from build123d import *

# Parameters (mm, degrees)
BOSS_EXTRUDE1_DEPTH             = 25
SKETCH2_R                       = 1.55
CUT_EXTRUDE1_DEPTH              = 17.55
BOSS_EXTRUDE2_REACH             = 68.8
BOSS_EXTRUDE2_DIRECTION_2_DEPTH = 30
CUT_EXTRUDE2_REACH              = 80.634
CUT_EXTRUDE2_END_RADIUS         = 15.55
SKETCH7_R                       = 1.55


with BuildPart() as part:
    # Sketch1 → Boss-Extrude1 (new, symmetric)
    with BuildSketch(Plane.XY):
        with BuildLine():
            Line((-20.55, 17.55), (-20.55, 0))
            Line((-20.55, 0), (20.55, 0))
            Line((20.55, 0), (20.55, 17.55))
            Line((20.55, 17.55), (12.55, 17.55))
            ThreePointArc((12.55, 17.55), (0, 5), (-12.55, 17.55))
            Line((-12.55, 17.55), (-20.55, 17.55))
        make_face()
    extrude(amount=BOSS_EXTRUDE1_DEPTH, both=True)

    # Sketch2 → Cut-Extrude1 (cut)
    with BuildSketch(Plane(origin=(0, 17.55, 0), x_dir=(1, 0, 0), z_dir=(0, 1, 0))):
        with Locations(Location((-16.55, 15, 0), (0, 0, 270))):
            Circle(SKETCH2_R)
        with Locations(Location((16.55, 15, 0), (0, 0, 270))):
            Circle(SKETCH2_R)
        with Locations(Location((16.55, -15, 0), (0, 0, 270))):
            Circle(SKETCH2_R)
        with Locations(Location((-16.55, -15, 0), (0, 0, 270))):
            Circle(SKETCH2_R)
    extrude(amount=-CUT_EXTRUDE1_DEPTH, mode=Mode.SUBTRACT)

    # Boss-Extrude2: up to this plane
    boss_extrude2_end = Plane(origin=(20.55, 0, 25), z_dir=(-1, 0, 0))
    # Sketch5 → Boss-Extrude2 (add, up to the surface)
    with BuildSketch(Plane(origin=(28.704083189, 0, 16.572310156), x_dir=(0.500000000000001, 0, -0.8660254037844382), z_dir=(0.866025403784438, 0, 0.5000000000000009)), mode=Mode.PRIVATE) as boss_extrude2_sk1:
        with BuildLine():
            Line((-5.334622532, 17.55), (-2.314823147, 17.55))
            ThreePointArc((-2.314823147, 17.55), (10.235176853, 5), (22.785176853, 17.55))
            Line((22.785176853, 17.55), (25.765377468, 17.55))
            ThreePointArc((25.765377468, 17.55), (10.215377468, 2), (-5.334622532, 17.55))
        make_face()
    boss_extrude2_tool1 = split(extrude(boss_extrude2_sk1.sketch, amount=-BOSS_EXTRUDE2_REACH, mode=Mode.PRIVATE), bisect_by=boss_extrude2_end, keep=Keep.BOTH, mode=Mode.PRIVATE)
    add(boss_extrude2_tool1.solids().sort_by_distance((33.811772, 2.347709, 7.725534))[0])

    # Sketch5 → Boss-Extrude2 direction 2 (add)
    with BuildSketch(Plane(origin=(28.704083189, 0, 16.572310156), x_dir=(0.500000000000001, 0, -0.8660254037844382), z_dir=(0.866025403784438, 0, 0.5000000000000009))):
        with BuildLine():
            Line((-5.334622532, 17.55), (-2.314823147, 17.55))
            ThreePointArc((-2.314823147, 17.55), (10.235176853, 5), (22.785176853, 17.55))
            Line((22.785176853, 17.55), (25.765377468, 17.55))
            ThreePointArc((25.765377468, 17.55), (10.215377468, 2), (-5.334622532, 17.55))
        make_face()
    extrude(amount=BOSS_EXTRUDE2_DIRECTION_2_DEPTH)

    # Cut-Extrude2: up to this cylinder (the profile starts inside it)
    cut_extrude2_end = Plane(origin=(46.802153231, 17.55, 15.225533904), z_dir=(-0.8660254037844382, 0, -0.500000000000001)) * Cylinder(CUT_EXTRUDE2_END_RADIUS, 193.368, mode=Mode.PRIVATE)
    # Sketch7 → Cut-Extrude2 (cut, up to the surface)
    with BuildSketch(Plane(origin=(0, 17.55, 0), x_dir=(1, 0, 0), z_dir=(0, 1, 0)), mode=Mode.PRIVATE) as cut_extrude2_sk1:
        with Locations(Location((46.812052672, -15.20838699, 0), (0, 0, 180))):
            Circle(SKETCH7_R)
    cut_extrude2_tool1 = extrude(cut_extrude2_sk1.sketch, amount=-CUT_EXTRUDE2_REACH, mode=Mode.PRIVATE) & cut_extrude2_end
    add(cut_extrude2_tool1.solids().sort_by_distance((46.812053, 17.55, 15.208387))[0], mode=Mode.SUBTRACT)


solid = part.part
Work out the finished part from the listing and answer in its coordinate system (mm). A direction names the side the tool comes from. Give positions to 0.01 mm unless a question says otherwise; leave off trailing zeros. Loops run counter-clockwise (first coordinate to the right, second up) from the corner with the lowest first, then second, coordinate; pieces in that order, holes last. Notation, with made-up numbers: (53.25, 87.5) - (104.25, 87.5) arc R29 ccw to (104.25, 114.5) - close; hole circle Ø1 at (24.25, -27.75). An arc over 180 degrees is marked (long way). Answer in a Markdown table with one row per item. Add a question column.
Q1. Each of these flat-tipped pins is pushed along its axis until it touches: P1, Ø8, axis at x = 45, y = 6.5, coming from the +Z side; P2, Ø3, axis at x = 16.55, z = -15, coming from the -Y side; P3, Ø4, axis at x = -6.5, y = 7, coming from the +Z side; P4, Ø5, axis at x = 46.81, z = 15.21, coming from the +Y side. Where does it stop, or does it pass through?
Q2. The part is cut by section B-B (x = -16.55). Determine the outline of the cut face in (y, z).
Q3. The part is cut by section A-A (y = 10.5). Determine the outline of the cut face in (x, z).
Q4. The part is cut by section C-C (y = 14.5). Determine the outline of the cut face in (x, z), and give its area (3 significant figures).
Q5. A tool of negligible diameter and unlimited length cuts with its end or side. For faces 1 (the flat face through (20.55, 1, 0)), 2 (the flat face through (0, 3, 25)), 3 (the cylindrical face through (-17.49, 8.9, 13.77)), from which of +Z, -Z, +X, -X, +Y, -Y can it reach the whole face along a straight path? Write none if from no direction.
Q6. Determine the mould class of faces 4 (the cylindrical face through (-16.48, 8.9, -16.55)), 5 (the flat face through (-20.55, 9, 0)), 6 (the flat face through (20, 17.55, 2)) for opening direction X: released by +X, released by -X, zero draft, split by the parting line, or undercut.
Q7. The part is cut by section D-D (x = 0). Determine the outline of the cut face in (y, z).
Q8. Consider line 1 along X through (y, z) = (9.25, -15); line 2 along X through (y, z) = (8, 15); line 3 along X through (y, z) = (1.5, 19.5). Determine where each line is inside the solid, lowest interval first.
Solution:
| question | item | result |
|---|---|---|
| 1 | P1 | stops at z = 31.08 |
| 1 | P2 | passes through |
| 1 | P3 | stops at z = 25 |
| 1 | P4 | stops at y = 5.25 |
| 2 | outline | (0, -25) - (17.55, -25) - (17.55, -16.55) - (0, -16.55) - close; (0, -13.45) - (17.55, -13.45) - (17.55, 13.45) - (0, 13.45) - close; (0, 16.55) - (17.55, 16.55) - (17.55, 25) - (0, 25) - close |
| 3 | outline | (-20.55, -25) - (-10.38, -25) - (-10.38, 25) - (-20.55, 25) - close; (10.38, -25) - (20.55, -25) - (20.55, -15.94) - (66.72, 10.72) - (64.99, 13.72) - (20.55, -11.94) - (20.55, 12.03) - (54.61, 31.7) - (52.86, 34.73) - (20.55, 16.07) - (20.55, 25) - (10.38, 25) - close; hole circle Ø3.1 at (-16.55, -15); hole circle Ø3.1 at (-16.55, 15); hole circle Ø3.1 at (16.55, -15); hole circle Ø3.1 at (16.55, 15) |
| 4 | outline | (-20.55, -25) - (-12.17, -25) - (-12.17, 25) - (-20.55, 25) - close; (12.17, -25) - (20.55, -25) - (20.55, -17.54) - (67.42, 9.52) - (65.89, 12.17) - (20.55, -14.01) - (20.55, 14.1) - (53.72, 33.25) - (52.17, 35.93) - (20.55, 17.68) - (20.55, 25) - (12.17, 25) - close; hole circle Ø3.1 at (-16.55, -15); hole circle Ø3.1 at (-16.55, 15); hole circle Ø3.1 at (16.55, -15); hole circle Ø3.1 at (16.55, 15) |
| 4 | area | 1,090 mm² |
| 5 | face 1 | -Y |
| 5 | face 2 | +Z, -X, +Y, -Y |
| 5 | face 3 | +Y, -Y |
| 6 | face 4 | undercut |
| 6 | face 5 | released by -X |
| 6 | face 6 | zero draft |
| 7 | outline | (0, -25) - (5, -25) - (5, 25) - (0, 25) - close |
| 8 | line 1 | x = -20.55 to -18.1, -15 to -9.41, 9.41 to 15, 18.1 to 20.75 |
| 8 | line 2 | x = -20.55 to -18.1, -15 to -8.14, 8.14 to 15, 18.1 to 20.55, 21.87 to 30.17, 62.74 to 64.25 |
| 8 | line 3 | x = -20.55 to 20.55 |
